from build123d import *

# Parameters (mm, degrees)
F0_W     = 62
F0_H     = 42
F0_R     = 1.55
F0_R_2   = 12.5
F1_DEPTH = 8
F2_W     = 5
F2_H     = 21
F3_DEPTH = 20
F4_R     = 1.55
F5_DEPTH = 25
F6_R     = 2.55
F7_DEPTH = 3


with BuildPart() as f1:
    # F0 (on Front) → F1 (new body)
    with BuildSketch(Plane.XZ):
        with Locations((31, 21)):
            Rectangle(F0_W, F0_H)
        with Locations((10, 8)):
            Circle(F0_R, mode=Mode.SUBTRACT)
        with Locations((25.697473, 5.4)):
            Circle(F0_R, mode=Mode.SUBTRACT)
        with Locations((56.897473, 5.4)):
            Circle(F0_R, mode=Mode.SUBTRACT)
        with Locations((10, 21)):
            Circle(F0_R, mode=Mode.SUBTRACT)
        with Locations((10, 34)):
            Circle(F0_R, mode=Mode.SUBTRACT)
        with Locations((25.697473, 36.6)):
            Circle(F0_R, mode=Mode.SUBTRACT)
        with Locations((41.297473, 21)):
            Circle(F0_R_2, mode=Mode.SUBTRACT)
        with Locations((56.897473, 36.6)):
            Circle(F0_R, mode=Mode.SUBTRACT)
    extrude(amount=F1_DEPTH)

    # F2 (on face) → F3 (join)
    with BuildSketch(Plane(origin=(0, 0, 0), x_dir=(-1, 0, 0), z_dir=(0, 1, 0))):
        with Locations((-22.5, 20.5)):
            Rectangle(F2_W, F2_H)
    extrude(amount=F3_DEPTH)

    # F4 (on face) → F5 (cut)
    with BuildSketch(Plane.YZ.offset(25)):
        with Locations((10, 28)):
            Circle(F4_R)
        with Locations((10, 13)):
            Circle(F4_R)
    extrude(amount=-F5_DEPTH, mode=Mode.SUBTRACT)

    # F6 (on face) → F7 (cut)
    with BuildSketch(Plane.YZ.offset(25)):
        with Locations((10, 28)):
            Circle(F6_R)
        with Locations((10, 13)):
            Circle(F6_R)
    extrude(amount=-F7_DEPTH, mode=Mode.SUBTRACT)


solid = f1.part
Can you work these out from the model? Positions are in its coordinate system, mm. A direction names the side the tool comes from. Give positions to 0.01 mm unless a question says otherwise; leave off trailing zeros. Loops run counter-clockwise (first coordinate to the right, second up) from the corner with the lowest first, then second, coordinate; pieces in that order, holes last. Notation, with made-up numbers: (53.5, 80) - (60.5, 80) arc R10 ccw to (60.5, 86) - close; hole circle Ø8 at (-22, 75.25). An arc over 180 degrees is marked (long way). Return JSON: item names as keys, results as strings.
1. For faces 4 (the face through (23.52, 9.67, 30.53)), 5 (the face through (20, 10, 20)), 6 (the face through (25, 10, 20)), which set-ups out of +Z, -Z, +X, -X, +Y, -Y let a thin tool reach every point of the face, with its end or its side?
Output values:
{"face 4": "+X", "face 5": "+Z, -Z, -X, +Y", "face 6": "+Z, -Z, +X, +Y"}
2. I want a section at C-C on x = 43.5. Please give me the cut outline in (y, z).
Output values:
{"outline": "(-8, 0) - (0, 0) - (0, 8.7) - (-8, 8.7) - close; (-8, 33.3) - (0, 33.3) - (0, 42) - (-8, 42) - close"}
3. If I drill on line 1 (Z direction, x = 22.85, y = 10); line 2 (Z direction, x = 21, y = 10); line 3 (Z direction, x = 10, y = -2.25), over which ranges is the centre line in solid material (lowest first)?
Output values:
{"line 1": "z = 10 to 10.45, 15.55 to 25.45, 30.55 to 31", "line 2": "z = 10 to 11.45, 14.55 to 26.45, 29.55 to 31", "line 3": "z = 0 to 6.45, 9.55 to 19.45, 22.55 to 32.45, 35.55 to 42"}
4. I'm going to push flat-ended pins straight in: pin 1 Ø4 at (y, z) = (9, 13.5) entering from +X; pin 2 Ø3 at (x, z) = (10, 8) entering from -Y; pin 3 Ø5 at (x, z) = (10, 33.5) entering from +Y; pin 4 Ø4 at (x, y) = (21.5, 15) entering from +Z. Where does each tip first touch, or does it pass through?
Output values:
{"pin 1": "stops at x = 25", "pin 2": "passes through", "pin 3": "stops at y = 0", "pin 4": "stops at z = 31"}
5. I want a section at B-B on x = 10. Please give me the cut outline in (y, z), and give its area (3 significant figures).
Output values:
{"outline": "(-8, 0) - (0, 0) - (0, 6.45) - (-8, 6.45) - close; (-8, 9.55) - (0, 9.55) - (0, 19.45) - (-8, 19.45) - close; (-8, 22.55) - (0, 22.55) - (0, 32.45) - (-8, 32.45) - close; (-8, 35.55) - (0, 35.55) - (0, 42) - (-8, 42) - close", "area": "262 mm²"}
6. We'd pull the mould along Y, two halves only. Please class faces 1 (the face through (22, 12, 28)), 2 (the face through (31, 0, 12)), 3 (the face through (31, -4, 0)): +Y half, -Y half, draft (parallel to the pull), parting line (faces both ways), or undercut.
Output values:
{"face 1": "undercut", "face 2": "+Y half", "face 3": "draft"}
7. I want a section at A-A on z = 36.6. Please give me the cut outline in (x, y), and give its area (3 significant figures).
Output values:
{"outline": "(0, -8) - (24.15, -8) - (24.15, 0) - (0, 0) - close; (27.25, -8) - (55.35, -8) - (55.35, 0) - (27.25, 0) - close; (58.45, -8) - (62, -8) - (62, 0) - (58.45, 0) - close", "area": "446 mm²"}
8. I want a section at D-D on z = 21. Please give me the cut outline in (x, y), and give its area (3 significant figures).
Output values:
{"outline": "(0, -8) - (8.45, -8) - (8.45, 0) - (0, 0) - close; (11.55, -8) - (28.8, -8) - (28.8, 0) - (25, 0) - (25, 20) - (20, 20) - (20, 0) - (11.55, 0) - close; (53.8, -8) - (62, -8) - (62, 0) - (53.8, 0) - close", "area": "371 mm²"}
